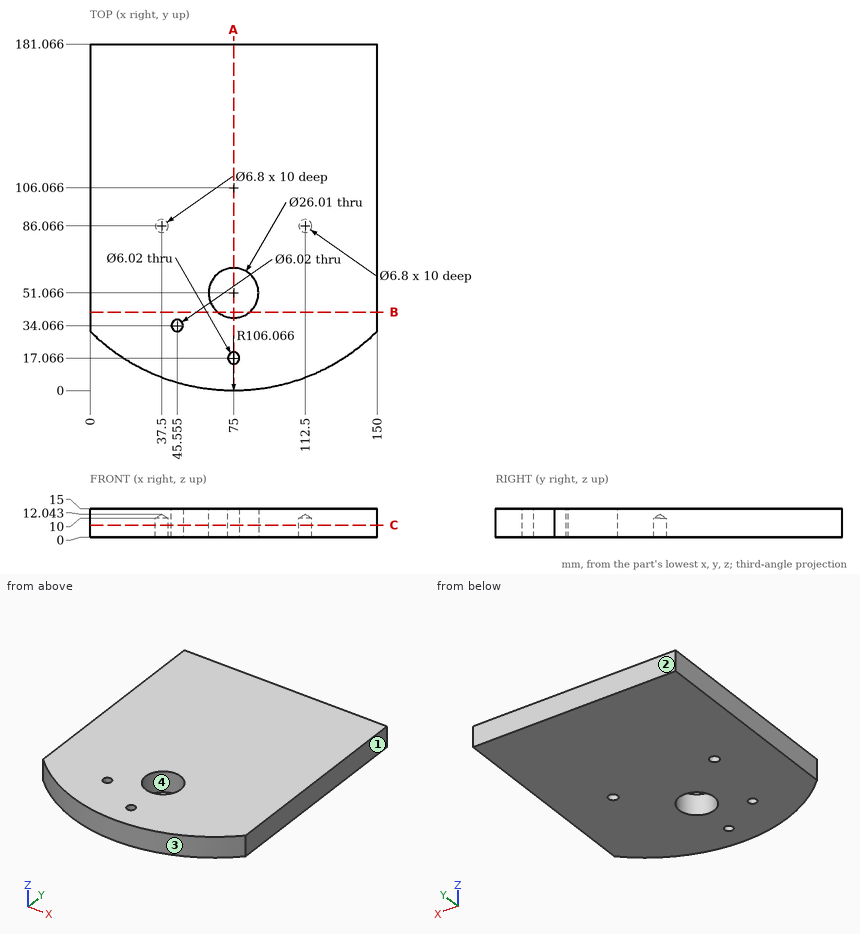
The drawing under review shows one solid part. Ordinate dimensions are in mm from its lowest x, y, z. Coordinates: 2 decimals unless noted, no trailing zeros. Order: outer loops, then holes, each group sorted by start corner. A loop starts at its lowest first (then second) coordinate and runs counter-clockwise, first axis right, second up. Notation, with made-up numbers: (78.5, -19.75) -> (93.5, -19.75) arc R22 ccw to (93.5, -4.75) -> close; hole circle Ø7 at (-35, 86). An arc over 180 degrees is marked (long way). Return JSON: item names as keys, results as strings.
1. We need section C-C on z = 6.5. Write out the cut boundary in (x, y) (3 decimals), and give its area (4 significant figures).
Answer block:
{"outline": "(0, 31.066) arc R106.066 ccw to (150, 31.066) -> (150, 181.066) -> (0, 181.066) -> close; hole circle Ø6.8 at (37.5, 86.066); hole circle Ø6.02 at (45.555, 34.066); hole circle Ø26.01 at (75, 51.066); hole circle Ø6.02 at (75, 17.066); hole circle Ø6.8 at (112.5, 86.066)", "area": "25,050 mm²"}
2. For line 1 (X direction, y = 87, z = 2.5); line 2 (X direction, y = 84.5, z = 10.5) (1 decimal); line 3 (X direction, y = 31.5, z = 12.75), list the stretches that pass through material, from the lowest coordinate up. Write a range as from..to.
Answer block:
{"line 1": "0..34.23, 40.77..109.23, 115.77..150", "line 2": "0..35.5, 39.5..110.5, 114.5..150", "line 3": "0..43.98, 47.13..150"}
3. We need section B-B on y = 41. Write out the cut boundary in (x, z), and give its area (3 significant figures).
Answer block:
{"outline": "(0, 0) -> (66.77, 0) -> (66.77, 15) -> (0, 15) -> close; (83.23, 0) -> (150, 0) -> (150, 15) -> (83.23, 15) -> close", "area": "2,000 mm²"}
4. We need section A-A on x = 75. Write out the cut boundary in (y, z).
Answer block:
{"outline": "(0, 0) -> (14.06, 0) -> (14.06, 15) -> (0, 15) -> close; (20.08, 0) -> (38.06, 0) -> (38.06, 15) -> (20.08, 15) -> close; (64.07, 0) -> (181.07, 0) -> (181.07, 15) -> (64.07, 15) -> close"}
5. For pin 1 Ø4 at (x, z) = (20, 13) entering from -Y, flat-tipped, find the tip position at first contact; note if it passes through.
Answer block:
{"pin 1": "y = 14.19"}
6. The part is to be moulded in two halves that separate along Y. For the marked faces 1, 2, 3 and 4, say which applies: +Y half, -Y half, draft (parallel to the pull), parting line (faces both ways), or undercut.
Answer block:
{"face 1": "draft", "face 2": "+Y half", "face 3": "-Y half", "face 4": "undercut"}
